```python
from build123d import *

# Parameters (mm, degrees)
BOSS_EXTRUDE1_DEPTH = 3
SKETCH2_R           = 2
CUT_EXTRUDE1_DEPTH  = 3


with BuildPart() as part:
    # Sketch1 → Boss-Extrude1 (new body)
    with BuildSketch(Plane(origin=(0, 0, 0), x_dir=(0, 0, -1), z_dir=(1, 0, 0))):
        Polygon((-9.832231839, 2.423101367), (-13.832231839, 2.423101367), (-13.832231839, -12.576898633), (-9.832231839, -12.576898633), (-9.832231839, -14.076898633), (16.167768161, -14.076898633), (16.167768161, -12.576898633), (20.167768161, -12.576898633), (20.167768161, 2.423101367), (16.167768161, 2.423101367), (16.167768161, 3.923101367), (-9.832231839, 3.923101367), align=None)
    extrude(amount=BOSS_EXTRUDE1_DEPTH)

    # Sketch2 → Cut-Extrude1 (cut)
    with BuildSketch(Plane.ZY):
        with Locations((-3.167768161, -5.076898633)):
            Circle(SKETCH2_R)
    extrude(amount=-CUT_EXTRUDE1_DEPTH, mode=Mode.SUBTRACT)


solid = part.part
```
Geometry check sheet. Reference: the model listing, model coordinates, mm. A direction names the side the tool comes from. Coordinates: 2 decimals unless noted, no trailing zeros. Order: outer loops, then holes, each group sorted by start corner. A loop starts at its lowest first (then second) coordinate and runs counter-clockwise, first axis right, second up. Notation, with made-up numbers: (-12.5, 88) - (23.5, 88) arc R29 ccw to (23.5, 124) - close; hole circle Ø4 at (15.5, 29). An arc over 180 degrees is marked (long way). Answer in a Markdown table with one row per item. Add a question column.
1. Access from +Z, -Z, +X, -X, +Y, -Y to the whole of each face (thin tool, end or side, straight path). Record for faces 1 (the face through (1, 2.423, -18)), 2 (the face through (1, -13, -16.168)), 3 (the face through (1, 2.423, 12)), 4 (the face through (1, -13, 9.832)).
2. Section check C-C (x = 0.35). Enter the section's corners in (y, z), plus the area to 3 significant figures.
3. Material ranges on L1, parallel to Z at x = 0.45, y = -3.75; L2, parallel to Z at x = 1.2, y = -3.5; L3, parallel to Y at x = 1.55, z = -16.5, recorded low to high. Write a range as [from, to].
4. Section check A-A (z = -2.5). Enter the section's corners in (x, y), plus the area to 3 significant figures.
5. Draft check along Z on faces 5 (the face through (1.48, -4.48, -1.26)), 6 (the face through (1, 3, -16.168)), 7 (the face through (0, -5, -7)), 8 (the face through (1, 3, 9.832)). Enter one of: +Z half, -Z half, draft (parallel to the pull), parting line (faces both ways), or undercut.
6. Gauge pin test, flat ends, axial feed: pin 1 Ø0.8 at (x, y) = (1.5, -13.5) entering from +Z; pin 2 Ø1.2 at (x, y) = (1, 3.5) entering from -Z; pin 3 Ø0.9 at (x, z) = (1.5, 12.5) entering from -Y. Record the tip position at first contact, or that the pin passes through.
7. Section check B-B (y = -6). Enter the section's corners in (x, z), plus the area to 3 significant figures.
Data:
| question | item | result |
|---|---|---|
| 1 | face 1 | -Z, +X, -X, +Y |
| 1 | face 2 | -Z, +X, -X, -Y |
| 1 | face 3 | +Z, +X, -X, +Y |
| 1 | face 4 | +Z, +X, -X, -Y |
| 2 | outline | (-14.08, -16.17) - (-12.58, -16.17) - (-12.58, -20.17) - (2.42, -20.17) - (2.42, -16.17) - (3.92, -16.17) - (3.92, 9.83) - (2.42, 9.83) - (2.42, 13.83) - (-12.58, 13.83) - (-12.58, 9.83) - (-14.08, 9.83) - close; hole circle Ø4 at (-5.08, -3.17) |
| 2 | area | 575 mm² |
| 3 | L1 | z = [-20.17, -4.66], [-1.67, 13.83] |
| 3 | L2 | z = [-20.17, -4.4], [-1.94, 13.83] |
| 3 | L3 | y = [-12.58, 2.42] |
| 4 | outline | (0, -14.08) - (3, -14.08) - (3, -6.96) - (0, -6.96) - close; (0, -3.19) - (3, -3.19) - (3, 3.92) - (0, 3.92) - close |
| 4 | area | 42.7 mm² |
| 5 | face 5 | undercut |
| 5 | face 6 | -Z half |
| 5 | face 7 | draft |
| 5 | face 8 | +Z half |
| 6 | pin 1 | stops at z = 9.83 |
| 6 | pin 2 | stops at z = -16.17 |
| 6 | pin 3 | stops at y = -12.58 |
| 7 | outline | (0, -20.17) - (3, -20.17) - (3, -4.94) - (0, -4.94) - close; (0, -1.39) - (3, -1.39) - (3, 13.83) - (0, 13.83) - close |
| 7 | area | 91.4 mm² |
